For this review, take the finished solid that the model builds, in its own axes (mm). Round coordinates to 2 decimals unless told otherwise and drop trailing zeros. Order: outer loops, then holes, each group sorted by start corner. A loop starts at its lowest first (then second) coordinate and runs counter-clockwise, first axis right, second up.
from build123d import *

# Parameters (mm, degrees)
SKETCH_1_R          = 32.5
SKETCH_1_R_2        = 13.025
EXTRUDE_1_DEPTH     = 4
EXTRUDE_START       = -4
EXTRUDE_2_DEPTH     = 4
SKETCH_4_R          = 1.6
CUT_EXTRUDE_1_DEPTH = 4
SKETCH_5_R          = 2.1
CUT_EXTRUDE_2_DEPTH = 4
SKETCH_6_R          = 1.6
CUT_EXTRUDE_3_DEPTH = 10
SKETCH_7_W          = 10
SKETCH_7_H          = 10
SKETCH_7_W_2        = 8
CUT_EXTRUDE_4_DEPTH = 10
FILLET_2_R          = 2
SKETCH_8_R          = 1.6
CUT_EXTRUDE_5_DEPTH = 10
EXTRUDE_4_DEPTH     = 4
FILLET_3_R          = 3
EXTRUDE_5_DEPTH     = 4
FILLET_4_R          = 2
CUT_EXTRUDE_6_DEPTH = 17
FILLET_5_R          = 2
SKETCH_14_R         = 1.6
CUT_EXTRUDE_7_DEPTH = 17
SKETCH_15_R         = 1.6
CUT_EXTRUDE_8_DEPTH = 10


with BuildPart() as part:
    # 草图1 → 凸台-拉伸1 (new body)
    with BuildSketch(Plane.XY):
        Circle(SKETCH_1_R)
        Circle(SKETCH_1_R_2, mode=Mode.SUBTRACT)
    extrude(amount=EXTRUDE_1_DEPTH)

    # 草图2 → 凸台-拉伸2 (add)
    with BuildSketch(Plane.XY.offset(4).offset(EXTRUDE_START)):
        with BuildLine():
            Line((-32.5, 0), (-32.5, -70))
            Line((-32.5, -70), (32.5, -70))
            Line((32.5, -70), (32.5, 0))
            ThreePointArc((32.5, 0), (0, -32.5), (-32.5, 0))
        make_face()
    extrude(amount=EXTRUDE_2_DEPTH)

    # 草图4 → 切除-拉伸1 (cut)
    with BuildSketch(Plane.XY.offset(4)):
        with Locations((0, 17.5)):
            Circle(SKETCH_4_R)
        with Locations((15.155444566, -8.75)):
            Circle(SKETCH_4_R)
        with Locations((-15.155444566, -8.75)):
            Circle(SKETCH_4_R)
    extrude(amount=-CUT_EXTRUDE_1_DEPTH, mode=Mode.SUBTRACT)

    # 草图5 → 切除-拉伸2 (cut)
    with BuildSketch(Plane.XY.offset(4)):
        with Locations((-20.5, -65)):
            Circle(SKETCH_5_R)
        with Locations((20.5, -65)):
            Circle(SKETCH_5_R)
    extrude(amount=-CUT_EXTRUDE_2_DEPTH, mode=Mode.SUBTRACT)

    # 草图6 → 切除-拉伸3 (cut)
    with BuildSketch(Plane(origin=(0, 0, 0), x_dir=(-1, 0, 0), z_dir=(0, 0, -1))):
        with Locations((-10, -50)):
            Circle(SKETCH_6_R)
        with Locations((10, -50)):
            Circle(SKETCH_6_R)
    extrude(amount=-CUT_EXTRUDE_3_DEPTH, mode=Mode.SUBTRACT)

    # 草图7 → 切除-拉伸4 (cut)
    with BuildSketch(Plane(origin=(0, 0, 0), x_dir=(-1, 0, 0), z_dir=(0, 0, -1))):
        with Locations((0, -38)):
            Rectangle(SKETCH_7_W, SKETCH_7_H)
        with Locations((12, -38)):
            Rectangle(SKETCH_7_W_2, SKETCH_7_H)
        with Locations((-12, -38)):
            Rectangle(SKETCH_7_W_2, SKETCH_7_H)
    extrude(amount=-CUT_EXTRUDE_4_DEPTH, mode=Mode.SUBTRACT)

    # 圆角2
    fillet_2_edges = [part.edges().sort_by_distance(p)[0] for p in [
        (32.5, -70, 2),
        (-8, -43, 2),
        (-8, -33, 2),
        (-16, -33, 2),
        (-16, -43, 2),
        (16, -43, 2),
        (16, -33, 2),
        (8, -33, 2),
        (8, -43, 2),
        (5, -43, 2),
        (5, -33, 2),
        (-5, -33, 2),
        (-5, -43, 2),
    ]]
    fillet(fillet_2_edges, radius=FILLET_2_R)

    # 草图8 → 切除-拉伸5 (cut)
    with BuildSketch(Plane.XY.offset(4)):
        with Locations((29.5, -58)):
            Circle(SKETCH_8_R)
        with Locations((29.5, -38)):
            Circle(SKETCH_8_R)
        with Locations((-29.5, -38)):
            Circle(SKETCH_8_R)
        with Locations((-29.5, -58)):
            Circle(SKETCH_8_R)
    extrude(amount=-CUT_EXTRUDE_5_DEPTH, mode=Mode.SUBTRACT)

    # 草图9 → 凸台-拉伸4 (add)
    with BuildSketch(Plane.XY.offset(4).offset(EXTRUDE_START)):
        with BuildLine():
            Line((11.665320616, 30.334308875), (19.746534697, 35))
            Line((19.746534697, 35), (22.961925006, 23))
            ThreePointArc((22.961925006, 23), (17.697727439, 27.258768194), (11.665320616, 30.334308875))
        make_face()
    extrude(amount=EXTRUDE_4_DEPTH)

    # 圆角3
    fillet_3_edges = [part.edges().sort_by_distance(p)[0] for p in [
        (22.961925006, 23, 2),
        (11.665320616, 30.334308875, 2),
        (19.746534697, 35, 2),
    ]]
    fillet(fillet_3_edges, radius=FILLET_3_R)

    # 草图11 → 凸台-拉伸5 (add)
    with BuildSketch(Plane(origin=(0, 0, 0), x_dir=(-1, 0, 0), z_dir=(0, 0, -1))):
        Polygon((32.5, 0), (62.5, -70), (32.5, -70), align=None)
    extrude(amount=-EXTRUDE_5_DEPTH)

    # 圆角4
    fillet_4_edges = [part.edges().sort_by_distance(p)[0] for p in [
        (-32.5, 0, 2),
        (-62.5, -70, 2),
    ]]
    fillet(fillet_4_edges, radius=FILLET_4_R)

    # 草图12 → 切除-拉伸6 (cut)
    with BuildSketch(Plane(origin=(0, 0, 0), x_dir=(-1, 0, 0), z_dir=(0, 0, -1))):
        with BuildLine():
            Line((-10.217621979, 18.916928955), (-11.540771679, 23.854990862))
            ThreePointArc((-11.540771679, 23.854990862), (-2.497822398, 26.38201818), (6.858704695, 25.597034397))
            Line((6.858704695, 25.597034397), (5.56460947, 20.767405265))
            ThreePointArc((5.56460947, 20.767405265), (-2.503736607, 21.353718716), (-10.217621979, 18.916928955))
        make_face()
        with BuildLine():
            Line((21.491352026, -0.609744277), (26.429413934, -1.932893978))
            ThreePointArc((26.429413934, -1.932893978), (24.096409146, -11.02783144), (18.738329701, -18.738329701))
            Line((18.738329701, -18.738329701), (15.202795796, -15.202795796))
            ThreePointArc((15.202795796, -15.202795796), (19.744731177, -8.508559852), (21.491352026, -0.609744277))
        make_face()
        with BuildLine():
            Line((-11.273730047, -18.307184678), (-14.888642254, -21.922096885))
            ThreePointArc((-14.888642254, -21.922096885), (-21.598586749, -15.354186741), (-25.597034397, -6.858704695))
            Line((-25.597034397, -6.858704695), (-20.767405265, -5.56460947))
            ThreePointArc((-20.767405265, -5.56460947), (-17.24099457, -12.845158864), (-11.273730047, -18.307184678))
        make_face()
    extrude(amount=-CUT_EXTRUDE_6_DEPTH, mode=Mode.SUBTRACT)

    # 圆角5
    fillet_5_edges = [part.edges().sort_by_distance(p)[0] for p in [
        (-15.202795796, -15.202795796, 2),
        (-21.491352026, -0.609744277, 2),
        (-26.429413934, -1.932893978, 2),
        (-18.738329701, -18.738329701, 2),
        (-5.56460947, 20.767405265, 2),
        (10.217621979, 18.916928955, 2),
        (11.540771679, 23.854990862, 2),
        (-6.858704695, 25.597034397, 2),
        (20.767405265, -5.56460947, 2),
        (11.273730047, -18.307184678, 2),
        (14.888642254, -21.922096885, 2),
        (25.597034397, -6.858704695, 2),
    ]]
    fillet(fillet_5_edges, radius=FILLET_5_R)

    # 草图14 → 切除-拉伸7 (cut)
    with BuildSketch(Plane(origin=(0, 0, 0), x_dir=(-1, 0, 0), z_dir=(0, 0, -1))):
        with Locations((33.458082183, -9.851298199)):
            Circle(SKETCH_14_R)
        with Locations((41.336468154, -28.234198799)):
            Circle(SKETCH_14_R)
        with Locations((49.214854126, -46.6170994)):
            Circle(SKETCH_14_R)
        with Locations((57.093240097, -65)):
            Circle(SKETCH_14_R)
        with BuildLine():
            Line((35.385724459, -27.042085352), (49.172899909, -59.212161403))
            ThreePointArc((49.172899909, -59.212161403), (48.122448446, -61.83829006), (45.496319789, -60.787838597))
            Line((45.496319789, -60.787838597), (31.709144338, -28.617762547))
            ThreePointArc((31.709144338, -28.617762547), (32.759595801, -25.991633889), (35.385724459, -27.042085352))
        make_face()
    extrude(amount=-CUT_EXTRUDE_7_DEPTH, mode=Mode.SUBTRACT)

    # 草图15 → 切除-拉伸8 (cut)
    with BuildSketch(Plane(origin=(0, 0, 0), x_dir=(-1, 0, 0), z_dir=(0, 0, -1))):
        with Locations((0, -27.5)):
            Circle(SKETCH_15_R)
        with Locations((-23.815698604, 13.75)):
            Circle(SKETCH_15_R)
        with Locations((23.815698604, 13.75)):
            Circle(SKETCH_15_R)
    extrude(amount=-CUT_EXTRUDE_8_DEPTH, mode=Mode.SUBTRACT)


solid = part.part
(1) Add section A-A on x = 0. Give the boundary of the cut face in (y, z) (3 decimals).
(2) Add section D-D on z = 2.5. Count the separate pieces of the cut face and the enclosed holes in it, plus the area to 3 significant figures.
(3) Add section C-C on y = -54. Give the boundary of the cut face in (x, z), plus the area to 3 significant figures.
(4) Wall thickness on L1, parallel to Y at x = 24, z = 3.85; L2, parallel to Y at x = 10, z = 1.5; L3, parallel to X at y = -3, z = 0.9: over which ranges is each line inside the solid? List them lowest first.
(5) Clearance check with flat-ended pins moving along their axes: P1, Ø2, axis at x = 1, z = 3, coming from the +Y side; P2, Ø2, axis at x = -11.5, z = 2, coming from the +Y side; P3, Ø2, axis at y = 14, z = 0.5, coming from the -X side. State where each tip first meets the part, or that it passes through.
(6) Add section B-B on x = -37. Give the boundary of the cut face in (y, z), plus the area to 3 significant figures.
(7) Draft analysis for pull direction X (two halves, no side actions). For faces 1 (the face through (0, -43, 2)), 2 (the face through (-5, -38, 2)), state which applies: pulls with the +X half, pulls with the -X half, needs draft (parallel to the pull), parting line crosses it, or undercut.
Here are the results:
1. outline: (-70, 0) - (-43, 0) - (-43, 4) - (-70, 4) - close; (-33, 0) - (-29.1, 0) - (-29.1, 4) - (-33, 4) - close; (-25.9, 0) - (-13.025, 0) - (-13.025, 4) - (-25.9, 4) - close; (13.025, 0) - (15.9, 0) - (15.9, 4) - (13.025, 4) - close; (19.1, 0) - (21.5, 0) - (21.5, 4) - (19.1, 4) - close; (26.5, 0) - (32.5, 0) - (32.5, 4) - (26.5, 4) - close
2. separate pieces: 1
2. enclosed holes: 26
2. area: 5,960 mm2
3. outline: (-55.64, 0) - (-46.94, 0) - (-46.94, 4) - (-55.64, 4) - close; (-42.59, 0) - (32.5, 0) - (32.5, 4) - (-42.59, 4) - close
3. area: 335 mm2
4. L1: y = -70 to -11.24, -6.48 to 12.16, 15.34 to 21.91
4. L2: y = -70 to -51.6, -48.4 to -43, -33 to -8.35, 8.35 to 20.07, 24.54 to 30.92
4. L3: x = -33.79 to -26.21, -21.29 to -12.67, 12.67 to 32.5
5. P1: stops at y = 32.5
5. P2: stops at y = 30.76
5. P3: stops at x = -29.79
6. outline: (-70, 0) - (-40.96, 0) - (-40.96, 4) - (-70, 4) - close; (-30.81, 0) - (-10.5, 0) - (-10.5, 4) - (-30.81, 4) - close
6. area: 197 mm2
7. face 1: undercut
7. face 2: undercut
